The model under review builds one solid part; all positions refer to its coordinate system, in mm. A direction names the side the tool comes from. Round coordinates to 2 decimals unless told otherwise and drop trailing zeros. Loops run counter-clockwise (first coordinate to the right, second up) from the corner with the lowest first, then second, coordinate; pieces in that order, holes last. Notation, with made-up numbers: M -3.5,49.5 L 23.5,49.5 A18 ccw 23.5,70.5 Z; hole C -27.75,-26 d7. An arc over 180 degrees is marked long. Answer as a JSON object with one key per item and string values. Group by question number.
Item 1: Consider section A-A (x = 45.5). Give the boundary of the cut face in (y, z), and give its area (3 significant figures).
Item 2: Consider section B-B (y = 13.75). Give the boundary of the cut face in (x, z).
Item 3: To check wall thickness, follow line 1 (Z direction, x = 28, y = 11.5); line 2 (Y direction, x = 29, z = -3). State the ranges of each line that lie inside material, in increasing order.
Item 4: Consider section C-C (z = 88). Give the boundary of the cut face in (x, y).
Item 5: Tool access review of faces 4 (the face through (85, 9, 15)), 5 (the face through (-60, 2, 0)), 6 (the face through (1, 10, 14)), 7 (the face through (60, 2, 30)), 8 (the face through (60, 0, 15)): name each direction out of +Z, -Z, +X, -X, +Y, -Y from which nothing blocks a thin tool from reaching the whole face with its end or side.
Item 6: Insertion check: P1, Ø1.5, axis at y = 1, z = 10.5, coming from the -X side; P2, Ø2.5, axis at y = 1, z = 16, coming from the +X side; P3, Ø1.5, axis at y = 5, z = 15.5, coming from the +X side; P4, Ø3.5, axis at y = 5, z = 17, coming from the +X side. Each pin has a flat end and moves straight along its axis. Give the tip position at first contact, or say it passes through.
Item 7: The part is to be moulded in two halves that separate along Z. For faces 1 (the face through (-1, 20, -78)), 2 (the face through (-1, 15, -75)), 3 (the face through (1, 13, -80)), say which applies: +Z half, -Z half, draft (parallel to the pull), parting line (faces both ways), or undercut.
```python
from build123d import *

# Parameters (mm, degrees)
EXTRUDE_1_DEPTH   = 30
EXTRUDE_1_2_DEPTH = 30
EXTRUDE_2_DEPTH   = 4
EXTRUDE_3_DEPTH   = 10


with BuildPart() as part:
    # Sketch 1 → Extrude 1 (new body)
    with BuildSketch(Plane.XY):
        Polygon((-55, 0), (-55, 3), (-57.5, 3), (-57.5, 6), (-62.5, 6), (-62.5, 3), (-65, 3), (-65, 0), align=None)
    extrude(amount=EXTRUDE_1_DEPTH)



with BuildPart() as body_2:
    # Sketch 1 → Extrude 1 2 (new body)
    with BuildSketch(Plane.XY):
        Polygon((65, 0), (55, 0), (55, 3), (57.5, 3), (57.5, 6), (62.5, 6), (62.5, 3), (65, 3), align=None)
    extrude(amount=EXTRUDE_1_2_DEPTH)


with BuildPart() as part_1:
    add(part.part)

    add(body_2.part)  # Extrude 2 merges body 2
    # Sketch 2 → Extrude 2 (add)
    with BuildSketch(Plane(origin=(0, 6, 0), x_dir=(1, 0, 0), z_dir=(0, 1, 0))):
        Polygon((0, -110), (-85, -110), (-85, 80), (85, 80), (85, -110), align=None)
    extrude(amount=EXTRUDE_2_DEPTH)

    # Sketch 3 → Extrude 3 (add)
    with BuildSketch(Plane(origin=(0, 10, 0), x_dir=(1, 0, 0), z_dir=(0, 1, 0))):
        Polygon((-85, 80), (-85, 75), (80, 75), (85, 75), (85, 80), align=None)
        Polygon((80, -105), (-85, -105), (-85, -110), (85, -110), (85, -105), align=None)
    extrude(amount=EXTRUDE_3_DEPTH)


solid = part_1.part
```
Geometry results:
{
 "1": {"outline": "M 6,-80 L 20,-80 L 20,-75 L 10,-75 L 10,105 L 20,105 L 20,110 L 6,110 Z", "area": "860 mm^2"},
 "2": {"outline": "M -85,-80 L 85,-80 L 85,-75 L -85,-75 Z; M -85,105 L 85,105 L 85,110 L -85,110 Z"},
 "3": {"line 1": "z = -80 to -75, 105 to 110", "line 2": "y = 6 to 10"},
 "4": {"outline": "M -85,6 L 85,6 L 85,10 L -85,10 Z"},
 "5": {"face 4": "+Z, -Z, +X, +Y, -Y", "face 5": "-Z, +X, -X, -Y", "face 6": "+X, -X, +Y", "face 7": "+Z, +X, -X, -Y", "face 8": "+Z, -Z, +X, -X, -Y"},
 "6": {"P1": "stops at x = -65", "P2": "stops at x = 65", "P3": "stops at x = 62.5", "P4": "stops at x = 85"},
 "7": {"face 1": "draft", "face 2": "undercut", "face 3": "-Z half"}
}
